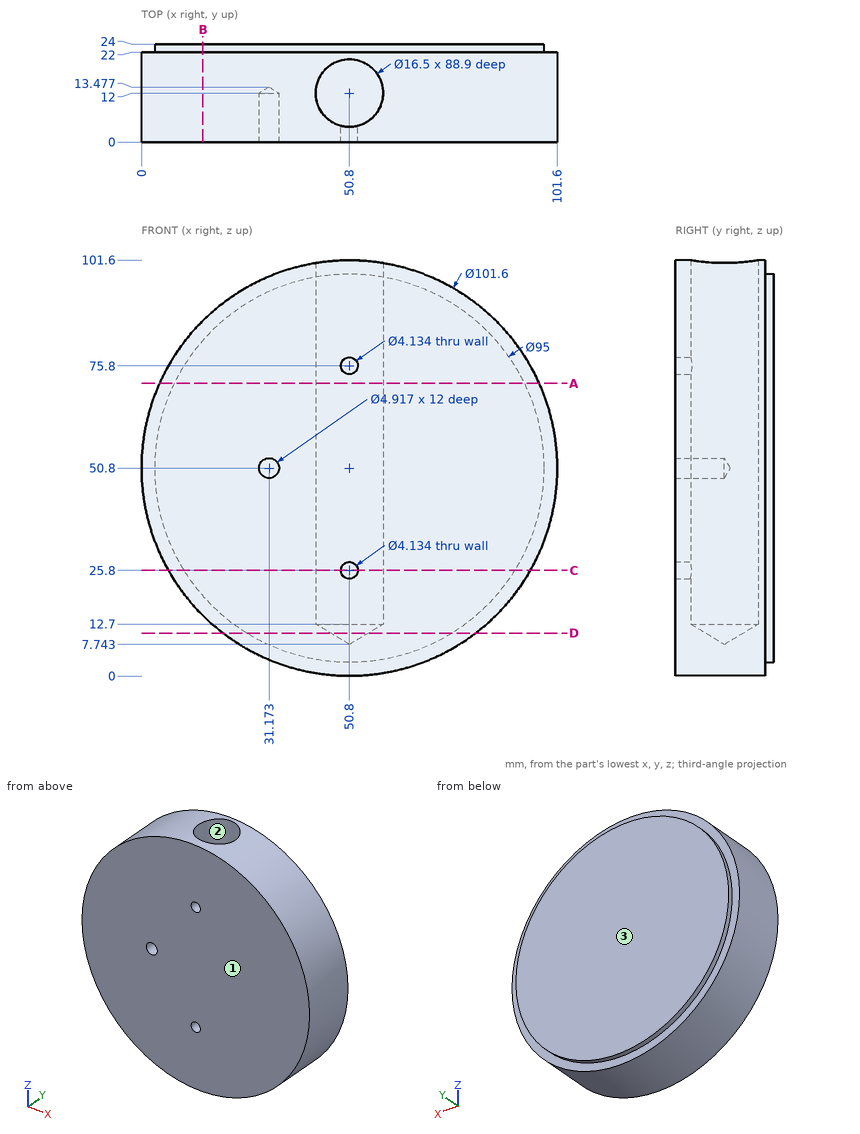
Study the drawing (mm; zero at the part's minimum x, y, z) and answer. Coordinates: 2 decimals unless noted, no trailing zeros. Write each loop counter-clockwise with the first axis right and the second up, starting at its lowest first coordinate (ties: lowest second). Pieces come first, ordered by that corner, then holes.
Q1. A cutting plane is placed at C-C, the plane z = 25.8. Give the vertices of the cut face in (x, y), then the cut area to 3 significant figures.
Q2. Determine the mould class of the marked faces 1, 2 and 3 for opening direction Y: released by +Y, released by -Y, zero draft, split by the parting line, or undercut.
Q3. A cutting plane is placed at A-A, the plane z = 71.5. Give the vertices of the cut face in (x, y), then the cut area to 3 significant figures.
Q4. A cutting plane is placed at D-D, the plane z = 10.5. Give the vertices of the cut face in (x, y).
Q5. Each of these flat-tipped pins is pushed along its axis until it touches: pin 1 Ø12 at (x, y) = (22, 12.5) entering from -Z; pin 2 Ø5 at (y, z) = (12, 72) entering from +X; pin 3 Ø1 at (x, y) = (84.5, 7.5) entering from -Z. Where does it stop, or does it pass through?
Q6. A cutting plane is placed at B-B, the plane x = 15. Give the vertices of the cut face in (y, z).
Q7. Find the intervals of material crossed by line 1 (Y direction, x = 12.5, z = 19.5); line 2 (X direction, y = 12, z = 67.5); line 3 (Y direction, x = 44.5, z = 84), in increasing order.
Findings below:
1. outline: (6.58, 0) - (48.73, 0) - (48.73, 4.01) arc R8.25 cw (long way) to (52.87, 4.01) - (52.87, 0) - (95.02, 0) - (95.02, 22) - (91.19, 22) - (91.19, 24) - (10.41, 24) - (10.41, 22) - (6.58, 22) - close
1. area: 1,880 mm2
2. face 1: released by -Y
2. face 2: undercut
2. face 3: released by +Y
3. outline: (4.41, 0) - (97.19, 0) - (97.19, 22) - (93.55, 22) - (93.55, 24) - (8.05, 24) - (8.05, 22) - (4.41, 22) - close; hole circle Ø16.5 at (50.8, 12)
3. area: 2,000 mm2
4. outline: (19.87, 0) - (81.73, 0) - (81.73, 22) - (75.94, 22) - (75.94, 24) - (25.66, 24) - (25.66, 22) - (19.87, 22) - close; hole circle Ø9.18 at (50.8, 12)
5. pin 1: stops at z = 5.4
5. pin 2: stops at x = 98.03
5. pin 3: stops at z = 12.35
6. outline: (0, 14.76) - (22, 14.76) - (22, 19.58) - (24, 19.58) - (24, 82.02) - (22, 82.02) - (22, 86.84) - (0, 86.84) - close
7. line 1: y = 0 to 22
7. line 2: x = 2.82 to 42.55, 59.05 to 98.78
7. line 3: y = 0 to 6.67, 17.33 to 24
